from build123d import *

# Parameters (mm, degrees)
SKETCH1_W           = 70
SKETCH1_H           = 70
BOSS_EXTRUDE1_DEPTH = 5
SKETCH2_R           = 12
SKETCH2_R_2         = 1.7
CUT_EXTRUDE6_DEPTH  = 50.749371855
CUT_EXTRUDE7_DEPTH  = 50.749371855


with BuildPart() as part:
    # Sketch1 → Boss-Extrude1 (new body)
    with BuildSketch(Plane.XY):
        Rectangle(SKETCH1_W, SKETCH1_H)
    extrude(amount=BOSS_EXTRUDE1_DEPTH)

    # Sketch2 → Cut-Extrude6 (cut, through all)
    with BuildSketch(Plane.XY.offset(5)):
        Circle(SKETCH2_R)
        with Locations((15.5, 15.112797807)):
            Circle(SKETCH2_R_2)
        with Locations((15.532292635, -15.887185373)):
            Circle(SKETCH2_R_2)
        with Locations(Location((-15.532292635, -15.887185373, 0), (0, 0, 180))):
            Circle(SKETCH2_R_2)
        with Locations(Location((-15.5, 15.112797807, 0), (0, 0, 180))):
            Circle(SKETCH2_R_2)
    extrude(amount=-CUT_EXTRUDE6_DEPTH, mode=Mode.SUBTRACT)

    # Sketch3 → Cut-Extrude7 (cut, through all)
    with BuildSketch(Plane.XY.offset(5)):
        with BuildLine():
            Line((-22, 9.22322481), (-22, -8.77677519))
            ThreePointArc((-22, -8.77677519), (-25, -11.77677519), (-28, -8.77677519))
            Line((-28, -8.77677519), (-28, 9.22322481))
            ThreePointArc((-28, 9.22322481), (-25, 12.22322481), (-22, 9.22322481))
        make_face()
        with BuildLine():
            Line((22, 9.22322481), (22, -8.77677519))
            ThreePointArc((22, -8.77677519), (25, -11.77677519), (28, -8.77677519))
            Line((28, -8.77677519), (28, 9.22322481))
            ThreePointArc((28, 9.22322481), (25, 12.22322481), (22, 9.22322481))
        make_face()
    extrude(amount=-CUT_EXTRUDE7_DEPTH, mode=Mode.SUBTRACT)


solid = part.part
Verification items for the finished model (mm, model axes). A direction names the side the tool comes from. Round coordinates to 2 decimals unless told otherwise and drop trailing zeros. Loops run counter-clockwise (first coordinate to the right, second up) from the corner with the lowest first, then second, coordinate; pieces in that order, holes last. Notation, with made-up numbers: (-38.5, 61) - (-33.5, 61) arc R16 ccw to (-33.5, 85) - close; hole circle Ø9 at (7, -4). An arc over 180 degrees is marked (long way). Use a Markdown table: item, result. Add a question column.
1. Section check A-A, the plane y = 0. Record the boundary of the cut face in (x, z), plus the area to 3 significant figures.
2. Gauge pin test, flat end, axial feed: pin 1 (2.5 mm diameter, centred on x = -15.53, y = -15.89, fed in from -Z). Record the tip position at first contact, or that the pin passes through.
3. Section check B-B, the plane x = 25. Record the boundary of the cut face in (y, z).
4. Release check for a two-part mould opening along Y. For faces 1 (the face through (0, 35, 2)), 2 (the face through (15, 0, 5)), 3 (the face through (0, -35, 2)), 4 (the face through (24.934, -11.776, 2.535)) record: released by +Y, released by -Y, zero draft, split by the parting line, or undercut.
5. Access from +Z, -Z, +X, -X, +Y, -Y to the whole of each face (thin tool, end or side, straight path). Record for faces 5 (the face through (15, 0, 0)), 6 (the face through (25.066, 12.222, 2.535)).
6. Thickness scan on probe 1 along Y at (x, z) = (-15.5, 3.9); probe 2 along Y at (x, z) = (15, 2.65); probe 3 along Y at (x, z) = (0, 2.3). Record the ranges inside material, lowest first. Write a range as [from, to].
7. Section check C-C, the plane x = -15.5. Record the boundary of the cut face in (y, z), plus the area to 3 significant figures.
8. Section check D-D, the plane z = 2.75. Record the boundary of the cut face in (x, y), plus the area to 3 significant figures.
Checks:
| question | item | result |
|---|---|---|
| 1 | outline | (-35, 0) - (-28, 0) - (-28, 5) - (-35, 5) - close; (-22, 0) - (-12, 0) - (-12, 5) - (-22, 5) - close; (12, 0) - (22, 0) - (22, 5) - (12, 5) - close; (28, 0) - (35, 0) - (35, 5) - (28, 5) - close |
| 1 | area | 170 mm^2 |
| 2 | pin 1 | passes through |
| 3 | outline | (-35, 0) - (-11.78, 0) - (-11.78, 5) - (-35, 5) - close; (12.22, 0) - (35, 0) - (35, 5) - (12.22, 5) - close |
| 4 | face 1 | released by +Y |
| 4 | face 2 | zero draft |
| 4 | face 3 | released by -Y |
| 4 | face 4 | undercut |
| 5 | face 5 | -Z, +X, -X, +Y, -Y |
| 5 | face 6 | +Z, -Z |
| 6 | probe 1 | y = [-35, -17.59], [-14.19, 13.41], [16.81, 35] |
| 6 | probe 2 | y = [-35, -17.5], [-14.27, 13.49], [16.74, 35] |
| 6 | probe 3 | y = [-35, -12], [12, 35] |
| 7 | outline | (-35, 0) - (-17.59, 0) - (-17.59, 5) - (-35, 5) - close; (-14.19, 0) - (13.41, 0) - (13.41, 5) - (-14.19, 5) - close; (16.81, 0) - (35, 0) - (35, 5) - (16.81, 5) - close |
| 7 | area | 316 mm^2 |
| 8 | outline | (-35, -35) - (35, -35) - (35, 35) - (-35, 35) - close; hole (-28, -8.78) arc R3 ccw to (-22, -8.78) - (-22, 9.22) arc R3 ccw to (-28, 9.22) - close; hole circle Ø3.4 at (-15.53, -15.89); hole circle Ø3.4 at (-15.5, 15.11); hole circle Ø24 at (0, 0); hole circle Ø3.4 at (15.5, 15.11); hole circle Ø3.4 at (15.53, -15.89); hole (22, -8.78) arc R3 ccw to (28, -8.78) - (28, 9.22) arc R3 ccw to (22, 9.22) - close |
| 8 | area | 4,140 mm^2 |
